from build123d import *

# Parameters (mm, degrees)
SKETCH3_R           = 7
BOSS_EXTRUDE1_DEPTH = 43


with BuildPart() as part:
    # Sketch3 → Boss-Extrude1 (new body)
    with BuildSketch(Plane.XY):
        with BuildLine():
            Line((-18.766263872, -12.144286576), (13.491947319, -12.144286576))
            ThreePointArc((13.491947319, -12.144286576), (15.646337823, -21.094858365), (20.497554358, -28.919168681))
            Line((20.497554358, -28.919168681), (25.709486961, -28.919168681))
            Line((25.709486961, -28.919168681), (54.709486961, 4.080831319))
            Line((54.709486961, 4.080831319), (54.709486961, 23.080831319))
            Line((54.709486961, 23.080831319), (48.896751189, 28.080831319))
            Line((48.896751189, 28.080831319), (24.896751189, 28.080831319))
            ThreePointArc((24.896751189, 28.080831319), (16.469153092, 18.865687614), (4.141554757, 16.872297921))
            Line((4.141554757, 16.872297921), (-12.778235346, 19.855713424))
            Line((-12.778235346, 19.855713424), (-19.778235346, 19.855713424))
            Line((-19.778235346, 19.855713424), (-26.290513039, 12.855713424))
            Line((-26.290513039, 12.855713424), (-26.290513039, -5.144286576))
            Line((-26.290513039, -5.144286576), (-18.766263872, -12.144286576))
        make_face()
        with Locations((-12.290513039, 3.855713424)):
            Circle(SKETCH3_R, mode=Mode.SUBTRACT)
    extrude(amount=BOSS_EXTRUDE1_DEPTH)


solid = part.part
Verification items for the finished model (mm, model axes). A direction names the side the tool comes from. Give positions to 0.01 mm unless a question says otherwise; leave off trailing zeros. Order: outer loops, then holes, each group sorted by start corner. A loop starts at its lowest first (then second) coordinate and runs counter-clockwise, first axis right, second up. Notation, with made-up numbers: (3.5, 11) -> (23.5, 11) arc R11 cw to (23.5, 16) -> close; hole circle Ø4 at (-38.75, -6.75). An arc over 180 degrees is marked (long way). Answer as CSV lines item,"result".
Q1. Scan lines: probe 1 along Y at (x, z) = (-13.5, 20); probe 2 along Y at (x, z) = (-16.5, 18.5); probe 3 along X at (y, z) = (5.5, 3). Record each from-to range of solid material in increasing order.
Solutions:
probe 1,"y = -12.14 to -3.04, 10.75 to 19.86"
probe 2,"y = -12.14 to -1.74, 9.45 to 19.86"
probe 3,"x = -26.29 to -19.09, -5.49 to 54.71"
Q2. Sectioned sample at B-B on y = 8.5. Record the cut outline in (x, z), plus the area to 3 significant figures.
Solutions:
outline,"(-26.29, 0) -> (-17.53, 0) -> (-17.53, 43) -> (-26.29, 43) -> close; (-7.05, 0) -> (54.71, 0) -> (54.71, 43) -> (-7.05, 43) -> close"
area,"3,030 mm²"
Q3. Sectioned sample at C-C on x = 47. Record the cut outline in (y, z).
Solutions:
outline,"(-4.69, 0) -> (28.08, 0) -> (28.08, 43) -> (-4.69, 43) -> close"
Q4. Sectioned sample at A-A on z = 33.5. Record the cut outline in (x, y), plus the area to 3 significant figures.
Solutions:
outline,"(-26.29, -5.14) -> (-18.77, -12.14) -> (13.49, -12.14) arc R29 ccw to (20.5, -28.92) -> (25.71, -28.92) -> (54.71, 4.08) -> (54.71, 23.08) -> (48.9, 28.08) -> (24.9, 28.08) arc R19 cw to (4.14, 16.87) -> (-12.78, 19.86) -> (-19.78, 19.86) -> (-26.29, 12.86) -> close; hole circle Ø14 at (-12.29, 3.86)"
area,"2,750 mm²"
Q5. Sectioned sample at D-D on y = -16. Record the cut outline in (x, z), plus the area to 3 significant figures.
Solutions:
outline,"(14.05, 0) -> (37.06, 0) -> (37.06, 43) -> (14.05, 43) -> close"
area,"989 mm²"
Q6. Access from +Z, -Z, +X, -X, +Y, -Y to the whole of each face (thin tool, end or side, straight path). Record for faces 1 (the flat face through (-3, -12.144, 21)), 2 (the flat face through (-26.291, 4, 21)), 3 (the flat face through (-4.2, 18.343, 21.199)).
Solutions:
face 1,"+Z, -Z, -X, -Y"
face 2,"+Z, -Z, -X, +Y, -Y"
face 3,"+Z, -Z, +Y"
Q7. Release check for a two-part mould opening along Y. For faces 4 (the flat face through (23, 6, 0)), 5 (the flat face through (-16, 19.856, 21)), 6 (the cylindrical face through (-19.284, 4.163, 21.199)) record: +Y half, -Y half, draft (parallel to the pull), parting line (faces both ways), or undercut.
Solutions:
face 4,"draft"
face 5,"+Y half"
face 6,"undercut"
Q8. Depth check by flat-ended pin: pin 1 (10 mm diameter, centred on x = -12, z = 5.5, fed in from +Y); pin 2 (1.5 mm diameter, centred on y = -10, z = 7.5, fed in from +X); pin 3 (3 mm diameter, centred on x = -4.5, z = 30.5, fed in from +Y). Enter the tip coordinate at first touch or a pass-through.
Solutions:
pin 1,"stops at y = 19.86"
pin 2,"stops at x = 42.99"
pin 3,"stops at y = 18.66"
